Geometry check sheet. Reference: the model listing, model coordinates, mm. Coordinates: 2 decimals unless noted, no trailing zeros. Order: outer loops, then holes, each group sorted by start corner. A loop starts at its lowest first (then second) coordinate and runs counter-clockwise, first axis right, second up. Notation, with made-up numbers: M 81,60.25 L 124,60.25 A12 ccw 124,64.25 Z; hole C -12.75,81 d4. An arc over 180 degrees is marked long. Use CSV: the item, a comma, the result in double quotes. Start each with the question number.
```python
from build123d import *

# Parameters (mm, degrees)
F0_R     = 50
F0_R_2   = 15
F1_DEPTH = 5


with BuildPart() as f1:
    # F0 (on Front) → F1 (new body, symmetric)
    with BuildSketch(Plane.XZ):
        Circle(F0_R)
        with Locations((-17.6335575688, -24.2705098312)):
            Circle(F0_R_2, mode=Mode.SUBTRACT)
        with Locations((17.6335575688, -24.2705098312)):
            Circle(F0_R_2, mode=Mode.SUBTRACT)
        with Locations((-28.5316954889, 9.2705098312)):
            Circle(F0_R_2, mode=Mode.SUBTRACT)
        with Locations((28.5316954889, 9.2705098312)):
            Circle(F0_R_2, mode=Mode.SUBTRACT)
        with Locations((0, 30)):
            Circle(F0_R_2, mode=Mode.SUBTRACT)
    extrude(amount=F1_DEPTH, both=True)


solid = f1.part
```
1) Gauge pin test, flat ends, axial feed: P1, Ø1.5, axis at y = 3.5, z = 11, coming from the +X side; P2, Ø24, axis at x = 0, z = 30, coming from the -Y side; P3, Ø3, axis at x = -9.5, y = -1.5, coming from the +Z side; P4, Ø1, axis at y = -3.5, z = -35.5, coming from the +X side. Record the tip position at first contact, or that the pin passes through.
2) Section check C-C on z = -19. Record the boundary of the cut face in (x, y), then the cut area to 3 significant figures.
3) Material ranges on line 1 along X through (y, z) = (1.5, -37.5); line 2 along Z through (x, y) = (0, -0.75); line 3 along Z through (x, y) = (-19.5, -3.5), recorded low to high.
4) Section check B-B on x = 0. Record the boundary of the cut face in (y, z).
5) Section check D-D on x = -30.5. Record the boundary of the cut face in (y, z), then the cut area to 3 significant figures.
6) Section check A-A on z = 30. Record the boundary of the cut face in (x, y).
7) Draft check along Z on faces 1 (the face through (-1, -5, 1)), 2 (the face through (47.69, -0.07, 15.02)), 3 (the face through (-30.484, 0.07, 24.143)), 4 (the face through (-3.78, 0.07, -30.02)). Enter one of: +Z half, -Z half, draft (parallel to the pull), parting line (faces both ways), or undercut.
Results are:
1,P1,"stops at x = 48.94"
1,P2,"passes through"
1,P3,"stops at z = 49.36"
1,P4,"stops at x = 35.71"
2,outline,"M -46.25,-5 L -31.68,-5 L -31.68,5 L -46.25,5 Z; M -3.59,-5 L 3.59,-5 L 3.59,5 L -3.59,5 Z; M 31.68,-5 L 46.25,-5 L 46.25,5 L 31.68,5 Z"
2,area,"363 mm²"
3,line 1,"x = -33.07 to -24.7, -10.56 to 10.56, 24.7 to 33.07"
3,line 2,"z = -50 to 15, 45 to 50"
3,line 3,"z = -46.04 to -39.15, -9.39 to -2.71, 21.25 to 46.04"
4,outline,"M -5,-50 L 5,-50 L 5,15 L -5,15 Z; M -5,45 L 5,45 L 5,50 L -5,50 Z"
5,outline,"M -5,-39.62 L 5,-39.62 L 5,-31.98 L -5,-31.98 Z; M -5,-16.56 L 5,-16.56 L 5,-5.6 L -5,-5.6 Z; M -5,24.14 L 5,24.14 L 5,39.62 L -5,39.62 Z"
5,area,"341 mm²"
6,outline,"M -40,-5 L -15,-5 L -15,5 L -40,5 Z; M 15,-5 L 40,-5 L 40,5 L 15,5 Z"
7,face 1,"draft"
7,face 2,"parting line"
7,face 3,"undercut"
7,face 4,"undercut"
